Check sheet for the modelled part. Datum: model origin and axes. Units: mm. Face numbers are marked on the shaded views. A direction names the side the tool comes from. Coordinates: 2 decimals unless noted, no trailing zeros. Loops run counter-clockwise (first coordinate to the right, second up) from the corner with the lowest first, then second, coordinate; pieces in that order, holes last. Notation, with made-up numbers: (74, 75) -> (83, 75) arc R5 cw to (83, 84) -> close; hole circle Ø7 at (17.5, 16). An arc over 180 degrees is marked (long way). Use one line per item in the form item = value.
from build123d import *

# Parameters (mm, degrees)
BOSS_EXTRUDE1_DEPTH = 4
CHAMFER2_SIZE       = 1
SKETCH4_R           = 2.5
BOSS_EXTRUDE3_DEPTH = 9


with BuildPart() as part:
    # Sketch2 → Boss-Extrude1 (new body)
    with BuildSketch(Plane(origin=(0, 0, 0), x_dir=(1, 0, 0), z_dir=(0, 1, 0))):
        Polygon((5.482188976, 1.810783632), (1.172909862, 5.653106738), (-4.309279114, 3.842323106), (-5.482188976, -1.810783632), (-1.172909862, -5.653106738), (4.309279114, -3.842323106), align=None)
    extrude(amount=BOSS_EXTRUDE1_DEPTH)

    # Chamfer2
    chamfer2_edges = [part.edges().sort_by_distance(p)[0] for p in [
        (-1.568184626, 4, -4.747714922),
        (-4.895734045, 4, -1.015769737),
        (-3.327549419, 4, 3.731945185),
        (1.568184626, 4, 4.747714922),
        (4.895734045, 4, 1.015769737),
        (3.327549419, 4, -3.731945185),
    ]]
    chamfer(chamfer2_edges, length=CHAMFER2_SIZE)

    # Sketch4 → Boss-Extrude3 (add)
    with BuildSketch(Plane.XZ):
        Circle(SKETCH4_R)
    extrude(amount=BOSS_EXTRUDE3_DEPTH)


solid = part.part
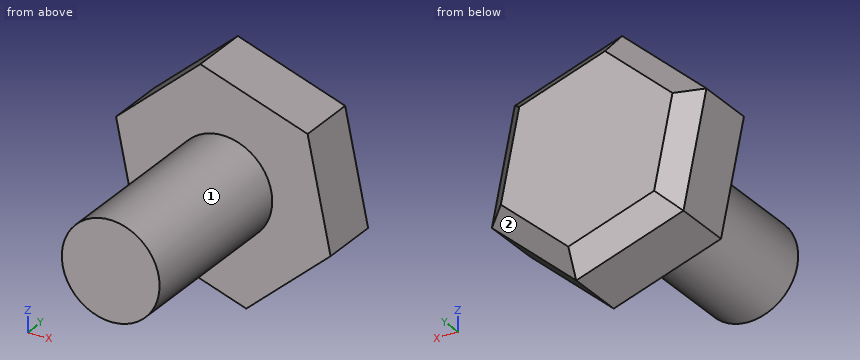
(1) Section check A-A, the plane x = -3.75. Record the boundary of the cut face in (y, z).
Established:
outline = (0, -4.03) -> (3, -4.03) -> (3.65, -3.34) -> (4, -1.62) -> (4, 2.02) -> (3, 3.36) -> (0, 3.36) -> close
(2) Section check D-D, the plane x = 0. Record the boundary of the cut face in (y, z).
Established:
outline = (-9, -2.5) -> (0, -2.5) -> (0, -5.27) -> (3, -5.27) -> (4, -4.21) -> (4, 4.21) -> (3, 5.27) -> (0, 5.27) -> (0, 2.5) -> (-9, 2.5) -> close
(3) Tool access check on the marked faces 1 and 2. Record the directions out of +Z, -Z, +X, -X, +Y, -Y that give a thin tool (end or side, any length) a straight path to the whole face; none if there is none.
Established:
face_1 = -Y
face_2 = -Z, +X, +Y
(4) Go/stop test with flat-tipped pins: P1, Ø4, axis at x = -2.5, y = 2.5, coming from the -Z side; P2, Ø1.5, axis at y = -5.5, z = -2.5, coming from the +X side. Record where each tip stops, or that it passes through.
Established:
P1 = -5.1
P2 = 1.79
(5) Section check B-B, the plane z = 0. Record the boundary of the cut face in (x, y), plus the area to 3 significant figures.
Established:
outline = (-5.11, 0) -> (-2.5, 0) -> (-2.5, -9) -> (2.5, -9) -> (2.5, 0) -> (5.11, 0) -> (5.11, 3) -> (4.09, 4) -> (-4.09, 4) -> (-5.11, 3) -> close
area = 84.8 mm²
(6) Scan lines: line 1 along Y through (x, z) = (-2.75, -1.5); line 2 along Y through (x, z) = (0, -4.5); line 3 along X through (y, z) = (-6.5, 1.5). Record each from-to range of solid material in increasing order.
Established:
line_1 = 0 to 4
line_2 = 0 to 3.73
line_3 = -2 to 2
(7) Section check C-C, the plane y = -1.5. Record the boundary of the cut face in (x, z).
Established:
outline = circle Ø5 at (0, 0)
